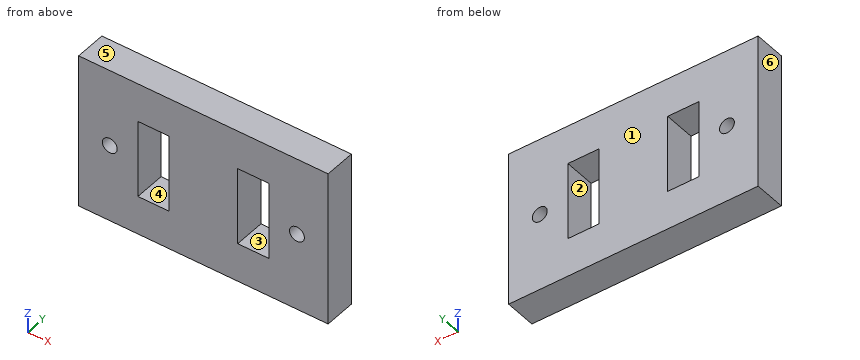
```python
from build123d import *

# Parameters (mm, degrees)
SKETCH1_W           = 80
SKETCH1_H           = 50
BOSS_EXTRUDE1_DEPTH = 10
SKETCH2_R           = 2.38125
CUT_EXTRUDE1_DEPTH  = 10
SKETCH3_W           = 10
SKETCH3_H           = 25
CUT_EXTRUDE2_DEPTH  = 10


with BuildPart() as part:
    # Sketch1 → Boss-Extrude1 (new body)
    with BuildSketch(Plane(origin=(0, 0, 0), x_dir=(1, 0, 0), z_dir=(0, 1, 0))):
        Rectangle(SKETCH1_W, SKETCH1_H)
    extrude(amount=BOSS_EXTRUDE1_DEPTH)

    # Sketch2 → Cut-Extrude1 (cut)
    with BuildSketch(Plane(origin=(0, 10, 0), x_dir=(1, 0, 0), z_dir=(0, 1, 0))):
        with Locations((-30, 0)):
            Circle(SKETCH2_R)
        with Locations((30, 0)):
            Circle(SKETCH2_R)
    extrude(amount=-CUT_EXTRUDE1_DEPTH, mode=Mode.SUBTRACT)

    # Sketch3 → Cut-Extrude2 (cut)
    with BuildSketch(Plane(origin=(0, 10, 0), x_dir=(1, 0, 0), z_dir=(0, 1, 0))):
        with Locations((-16, 0)):
            Rectangle(SKETCH3_W, SKETCH3_H)
        with Locations((16, 0)):
            Rectangle(SKETCH3_W, SKETCH3_H)
    extrude(amount=-CUT_EXTRUDE2_DEPTH, mode=Mode.SUBTRACT)


solid = part.part
```
Input: part model. Units: mm. Frame: model coordinates. Face numbers are marked on the shaded views. A direction names the side the tool comes from. Round coordinates to 2 decimals unless told otherwise and drop trailing zeros. Order: outer loops, then holes, each group sorted by start corner. A loop starts at its lowest first (then second) coordinate and runs counter-clockwise, first axis right, second up. Notation, with made-up numbers: (31, -28) - (74, -28) arc R16 ccw to (74, 1) - close; hole circle Ø6 at (25.25, -24). An arc over 180 degrees is marked (long way). Answer in a Markdown table with one row per item.
Item 1: Section query C-C (y = 9). Return the cut outline in (x, z).
Model answer:
| item | result |
|---|---|
| outline | (-40, -25) - (40, -25) - (40, 25) - (-40, 25) - close; hole circle Ø4.76 at (-30, 0); hole (-21, -12.5) - (-11, -12.5) - (-11, 12.5) - (-21, 12.5) - close; hole (11, -12.5) - (21, -12.5) - (21, 12.5) - (11, 12.5) - close; hole circle Ø4.76 at (30, 0) |
Item 2: Pin query (flat end, axial travel): pin 1 (7.5 mm diameter, centred on x = -30, z = 0, fed in from +Y). Return the tip coordinate at first contact, or that it passes through.
Model answer:
| item | result |
|---|---|
| pin 1 | stops at y = 10 |
Item 3: Mould query, pull axis X, two halves, no side actions, for the marked faces 3, 4, 5 and 6. Classes: released by +X, released by -X, zero draft, split by the parting line, or undercut.
Model answer:
| item | result |
|---|---|
| face 3 | undercut |
| face 4 | undercut |
| face 5 | zero draft |
| face 6 | released by -X |
Item 4: Line query: line 1 (X direction, y = 8.25, z = 11.5); line 2 (X direction, y = 2, z = 0); line 3 (Z direction, x = -30, y = 2.5). Output: solid intervals per line, ascending.
Model answer:
| item | result |
|---|---|
| line 1 | x = -40 to -21, -11 to 11, 21 to 40 |
| line 2 | x = -40 to -32.38, -27.62 to -21, -11 to 11, 21 to 27.62, 32.38 to 40 |
| line 3 | z = -25 to -2.38, 2.38 to 25 |
Item 5: Reachability of the marked faces 1 and 2 from +Z, -Z, +X, -X, +Y, -Y: full face, straight path, thin tool, end or side. Return the list, or none.
Model answer:
| item | result |
|---|---|
| face 1 | +Z, -Z, +X, -X, +Y |
| face 2 | +Y, -Y |
Item 6: Section query D-D (x = -15). Return the cut outline in (y, z).
Model answer:
| item | result |
|---|---|
| outline | (0, -25) - (10, -25) - (10, -12.5) - (0, -12.5) - close; (0, 12.5) - (10, 12.5) - (10, 25) - (0, 25) - close |
Item 7: Section query B-B (x = -30). Return the cut outline in (y, z), then the cut area to 3 significant figures.
Model answer:
| item | result |
|---|---|
| outline | (0, -25) - (10, -25) - (10, -2.38) - (0, -2.38) - close; (0, 2.38) - (10, 2.38) - (10, 25) - (0, 25) - close |
| area | 452 mm² |
Item 8: Section query A-A (z = 0). Return the cut outline in (x, y), then the cut area to 3 significant figures.
Model answer:
| item | result |
|---|---|
| outline | (-40, 0) - (-32.38, 0) - (-32.38, 10) - (-40, 10) - close; (-27.62, 0) - (-21, 0) - (-21, 10) - (-27.62, 10) - close; (-11, 0) - (11, 0) - (11, 10) - (-11, 10) - close; (21, 0) - (27.62, 0) - (27.62, 10) - (21, 10) - close; (32.38, 0) - (40, 0) - (40, 10) - (32.38, 10) - close |
| area | 505 mm² |
